Part print with two shaded views. Sizes in mm from the minimum x, y, z corner. A direction names the side the tool comes from. Round coordinates to 2 decimals unless told otherwise and drop trailing zeros. Order: outer loops, then holes, each group sorted by start corner. A loop starts at its lowest first (then second) coordinate and runs counter-clockwise, first axis right, second up. Notation, with made-up numbers: (9.5, 35.5) -> (18.5, 35.5) arc R23 cw to (18.5, 46.5) -> close; hole circle Ø11 at (81.5, 84.5). An arc over 180 degrees is marked (long way). Use a Markdown table: item, result. Add a question column.
Item 1: 3-axis set-ups, long thin cutter, end or side, ignore diameter. For the marked faces 1, 2 and 3: which of +Z, -Z, +X, -X, +Y, -Y reach the whole face in a straight line?
Item 2: Two-plate mould, pull along Y, no slides. Class the marked faces 4, 5 and 6: released by +Y, released by -Y, zero draft, split by the parting line, or undercut.
Item 3: Slice it at D-D, the plane x = 50.5. Give the cut face in (y, z).
Item 4: Probe L1, parallel to Y at x = 50, z = 30; L2, parallel to Z at x = 51, y = 35; L3, parallel to Z at x = 55, y = 40.5. List the from-to ranges inside material, lowest first.
Item 5: Slice it at B-B, the plane y = 35.4. Give the cut face in (x, z).
Item 6: Slice it at C-C, the plane z = 30. Give the cut face in (x, y).
Item 7: Slice it at A-A, the plane x = 30. Give the cut face in (y, z).
Item 8: Pin check, flat tips, straight feed: pin 1 (16.5 mm diameter, centred on y = 35.4, z = 30, fed in from +X); pin 2 (4 mm diameter, centred on x = 7, z = 12.5, fed in from -Y); pin 3 (15 mm diameter, centred on x = 30, y = 35.4, fed in from +Z). Stop position of each tip, or through.
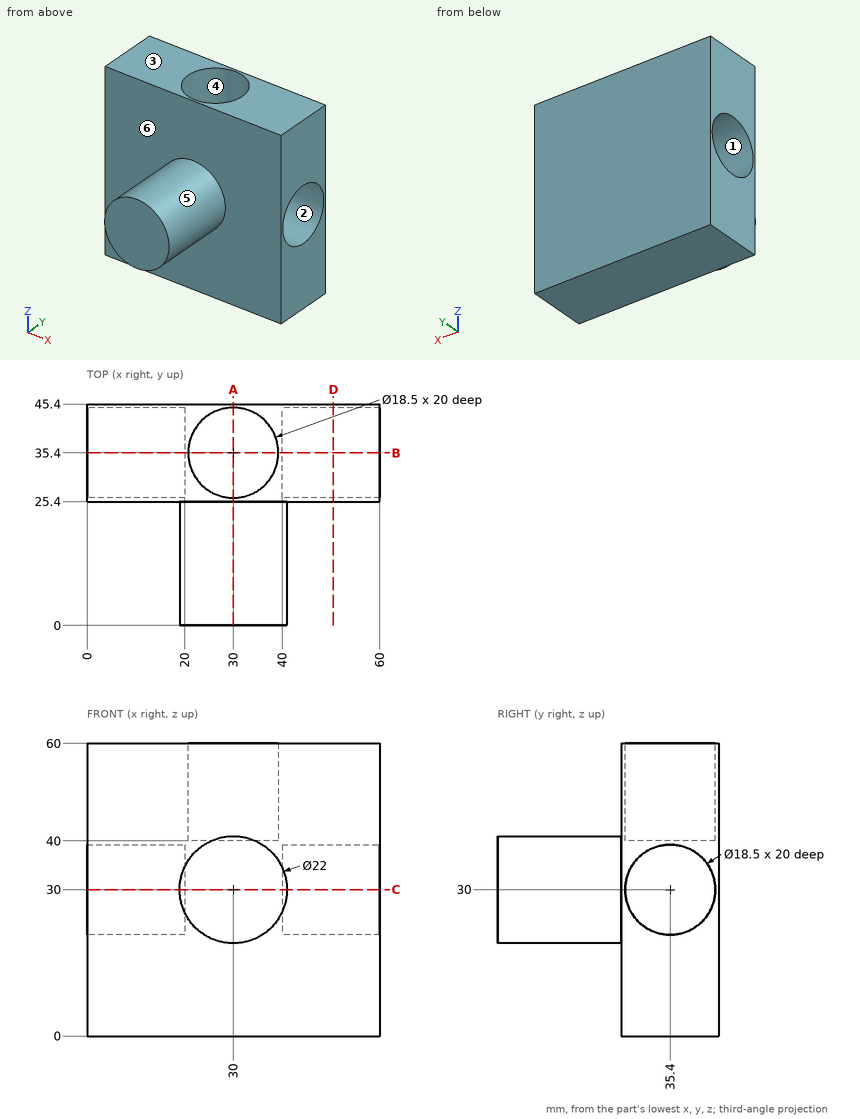
Check sheet entries:
| question | item | result |
|---|---|---|
| 1 | face 1 | -X |
| 1 | face 2 | +X |
| 1 | face 3 | +Z, +X, -X, +Y, -Y |
| 2 | face 4 | undercut |
| 2 | face 5 | zero draft |
| 2 | face 6 | released by -Y |
| 3 | outline | (25.4, 0) -> (45.4, 0) -> (45.4, 60) -> (25.4, 60) -> close; hole circle Ø18.5 at (35.4, 30) |
| 4 | L1 | 25.4 to 26.15, 44.65 to 45.4 |
| 4 | L2 | 0 to 20.76, 39.24 to 60 |
| 4 | L3 | 0 to 22.28, 37.72 to 60 |
| 5 | outline | (0, 0) -> (60, 0) -> (60, 20.75) -> (40, 20.75) -> (40, 39.25) -> (60, 39.25) -> (60, 60) -> (39.25, 60) -> (39.25, 40) -> (20.75, 40) -> (20.75, 60) -> (0, 60) -> (0, 39.25) -> (20, 39.25) -> (20, 20.75) -> (0, 20.75) -> close |
| 6 | outline | (0, 25.4) -> (19, 25.4) -> (19, 0) -> (41, 0) -> (41, 25.4) -> (60, 25.4) -> (60, 26.15) -> (40, 26.15) -> (40, 44.65) -> (60, 44.65) -> (60, 45.4) -> (0, 45.4) -> (0, 44.65) -> (20, 44.65) -> (20, 26.15) -> (0, 26.15) -> close |
| 7 | outline | (0, 19) -> (25.4, 19) -> (25.4, 0) -> (45.4, 0) -> (45.4, 60) -> (44.65, 60) -> (44.65, 40) -> (26.15, 40) -> (26.15, 60) -> (25.4, 60) -> (25.4, 41) -> (0, 41) -> close |
| 8 | pin 1 | x = 40 |
| 8 | pin 2 | y = 25.4 |
| 8 | pin 3 | z = 40 |
